```python
from build123d import *

# Parameters (mm, degrees)
F0_R     = 11
F1_DEPTH = 7
F2_R     = 9
F2_R_2   = 6
F3_DEPTH = 0.5
F4_R     = 3.95
F5_DEPTH = 7.001
F6_R     = 9
F6_R_2   = 6
F7_DEPTH = 0.5


with BuildPart() as f1:
    # F0 (on Top) → F1 (new body)
    with BuildSketch(Plane.XY):
        Circle(F0_R)
    extrude(amount=F1_DEPTH)

    # F2 (on face) → F3 (cut)
    with BuildSketch(Plane.XY.offset(7)):
        Circle(F2_R)
        Circle(F2_R_2, mode=Mode.SUBTRACT)
    extrude(amount=-F3_DEPTH, mode=Mode.SUBTRACT)

    # F4 (on face) → F5 (cut, through all)
    with BuildSketch(Plane.XY.offset(7)):
        Circle(F4_R)
    extrude(amount=-F5_DEPTH, mode=Mode.SUBTRACT)

    # F6 (on face) → F7 (cut)
    with BuildSketch(Plane.XY):
        Circle(F6_R)
        Circle(F6_R_2, mode=Mode.SUBTRACT)
    extrude(amount=F7_DEPTH, mode=Mode.SUBTRACT)


solid = f1.part
```
Could you check a few things on this model? Use its own coordinates, in mm. A direction names the side the tool comes from. Round coordinates to 2 decimals unless told otherwise and drop trailing zeros. Order: outer loops, then holes, each group sorted by start corner. A loop starts at its lowest first (then second) coordinate and runs counter-clockwise, first axis right, second up. Notation, with made-up numbers: M -2.5,86 L 8.5,86 A15 ccw 8.5,96 Z; hole C 1.5,28 d6. An arc over 180 degrees is marked long. One line per question, with ' | ' between items. Start each with the question number.
(1) Suppose I cut it at D-D on x = -7.5. List the corners of the cut face in (y, z) for me.
(2) For faces 1 (the face through (2, -6, 6.5)), 2 (the face through (2, -9, 0)), 3 (the face through (-5.994, 0.264, 0.246)), which set-ups out of +Z, -Z, +X, -X, +Y, -Y let a thin tool reach every point of the face, with its end or its side?
(3) Please list where these lines run through material, in increasing order: line 1 along Y through (x, z) = (0, 0.15); line 2 along Y through (x, z) = (0, 3); line 3 along Y through (x, z) = (-1.75, 5.25).
(4) Suppose I cut it at C-C on z = 2.75. List the corners of the cut face in (x, y) for me, then the cut area to 3 significant figures.
(5) For P1, Ø1.5, axis at y = -4, z = 6, coming from the +X side; P2, Ø6.5, axis at x = 0, y = 0, coming from the +Z side, each with a flat end and sliding along its axis, tell me the tip position at first contact or that it passes through.
(6) Suppose I cut it at A-A on y = 0. List the corners of the cut face in (x, z) for me.
(7) Thinking about a two-plate mould opening in X: for faces 4 (the face through (1, -4, 7)), 5 (the face through (-1.172, 8.923, 6.754)), 6 (the face through (-2.38, -10.74, 3.45)), which applies, +X half, -X half, draft (parallel to the pull), parting line (faces both ways), or undercut?
Geometry results:
1) outline: M -8.05,0 L -4.97,0 L -4.97,0.5 L 4.97,0.5 L 4.97,0 L 8.05,0 L 8.05,7 L 4.97,7 L 4.97,6.5 L -4.97,6.5 L -4.97,7 L -8.05,7 Z
2) face 1: +Z | face 2: -Z, +X, -X, +Y, -Y | face 3: -Z
3) line 1: -11 to -9, -6 to -3.95, 3.95 to 6, 9 to 11 | line 2: -11 to -3.95, 3.95 to 11 | line 3: -10.86 to -3.54, 3.54 to 10.86
4) outline: C 0,0 d22; hole C 0,0 d7.9 | area: 331 mm²
5) P1: x = 10.51 | P2: through
6) outline: M -11,0 L -9,0 L -9,0.5 L -6,0.5 L -6,0 L -3.95,0 L -3.95,7 L -6,7 L -6,6.5 L -9,6.5 L -9,7 L -11,7 Z; M 3.95,0 L 6,0 L 6,0.5 L 9,0.5 L 9,0 L 11,0 L 11,7 L 9,7 L 9,6.5 L 6,6.5 L 6,7 L 3.95,7 Z
7) face 4: draft | face 5: undercut | face 6: parting line
